Autodesk Fusion 360 part; units mm, degrees
sketch "Sketch1" plane through (0, 0, 0) normal (0, 1, 0) x (1, 0, 0)
  line L0 (0, 0) -> (0, -70)
  line L1 (0, -70) -> (60, -70)
  line L2 (60, -70) -> (60, -60)
  line L3 (60, -60) -> (55, -60)
  line L4 (55, -60) -> (45, 0)
  line L5 (45, 0) -> (0, 0)
  dimension "d1" = 90
  dimension "d2" = 70
  dimension "d3" = 45
  dimension "d4" = 60
  dimension "d5" = 5
  dimension "d6" = 10
revolve "Revolve1" add sketch "Sketch1" angle 360 about axis through (0, 0, 0) along (0, 0, 1)
shell "Shell1" thickness 5 removed faces 1 at (28.282, -12.1475, 70)
sketch "Sketch2" plane through (0, 0, 0) normal (1, 0, 0) x (0, 1, 0)
  line L0 (-7.5, 13) -> (7.5, 13)
  line L1 (7.5, 13) -> (7.5, 5)
  line L2 (7.5, 5) -> (-7.5, 5)
  line L3 (-7.5, 5) -> (-7.5, 13)
  dimension "d9" = 5
  dimension "d10" = 15
  dimension "d11" = 8
  dimension "d12" = 7.5
extrude "Extrude1" cut sketch "Sketch2" along normal through all
fillet "Fillet1" radius 1 4 edges at (42.642, 7.5, 5) (43.9954, 7.5, 13) (42.642, -7.5, 5) (43.9954, -7.5, 13)
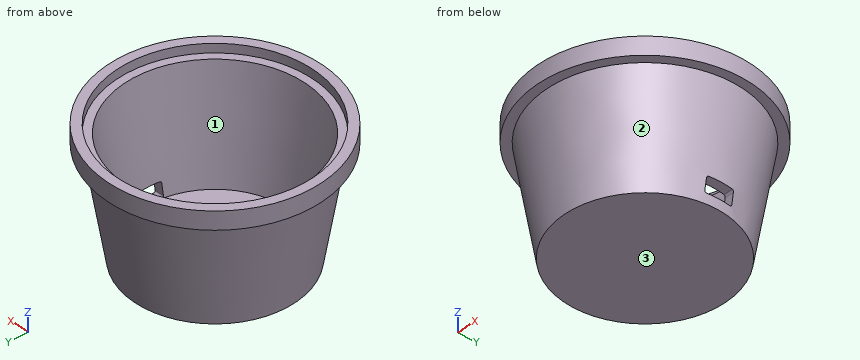
The model under review builds one solid part; all positions refer to its coordinate system, in mm. Face numbers are marked on the shaded views. Round coordinates to 2 decimals unless told otherwise and drop trailing zeros. Write each loop counter-clockwise with the first axis right and the second up, starting at its lowest first coordinate (ties: lowest second). Pieces come first, ordered by that corner, then holes. Notation, with made-up numbers: (74, 70.25) - (132, 70.25) arc R16 ccw to (132, 80.25) - close; hole circle Ø9 at (-32.5, -20.75). An arc over 180 degrees is marked (long way). One line per item, written item: value. Start each with the question number.
1. Consider section B-B on x = 0. Write out the cut boundary in (y, z), and give its area (3 significant figures).
2. Consider section A-A on y = 0. Write out the cut boundary in (x, z), and give its area (3 significant figures).
3. Consider section C-C on z = 51. Write out the cut boundary in (x, y), and give its area (3 significant figures).
4. To check wall thickness, follow L1, parallel to Y at x = 0, z = 67.35; L2, parallel to X at y = 11, z = 17.5; L3, parallel to X at y = 19.5, z = 33. State the ranges of each line that lie inside material, in increasing order. Write a range as from..to.
5. Clearance check with flat-ended pins moving along their axes: P1, Ø2, axis at x = -36, z = 31.5, coming from the +Y side; P2, Ø8, axis at y = -10, z = 33, coming from the -X side; P3, Ø5, axis at x = 43.5, z = 9.5, coming from the +Y side; P4, Ø1.7, axis at x = 44, y = -2.5, coming from the -Z side. State where each tip first meets the part, or that it passes through.
6. The part is to be moulded in two halves that separate along Y. For the marked faces 1, 2 and 3, say which applies: released by +Y, released by -Y, zero draft, split by the parting line, or undercut.
Checks:
1. outline: (-60, 60) - (-55, 60) - (-45, 0) - (45, 0) - (55, 60) - (60, 60) - (60, 70) - (55, 70) - (55, 65) - (50.76, 65) - (40.76, 5) - (-40.76, 5) - (-50.76, 65) - (-55, 65) - (-55, 70) - (-60, 70) - close
1. area: 1,160 mm^2
2. outline: (-60, 60) - (-55, 60) - (-45, 0) - (45, 0) - (45.83, 5) - (-40.76, 5) - (-50.76, 65) - (-55, 65) - (-55, 70) - (-60, 70) - close; (42.1, 13) - (47.17, 13) - (55, 60) - (60, 60) - (60, 70) - (55, 70) - (55, 65) - (50.76, 65) - close
2. area: 1,120 mm^2
3. outline: circle Ø107 at (0, 0); hole circle Ø96.86 at (0, 0)
3. area: 1,620 mm^2
4. L1: y = -60..-55, 55..60
4. L2: x = -46.64..-41.41, 41.41..46.64
4. L3: x = -46.58..-41.03, 41.03..46.58
5. P1: stops at y = 36.08
5. P2: stops at x = -50.47
5. P3: stops at y = 22.2
5. P4: stops at z = 0
6. face 1: undercut
6. face 2: split by the parting line
6. face 3: zero draft
